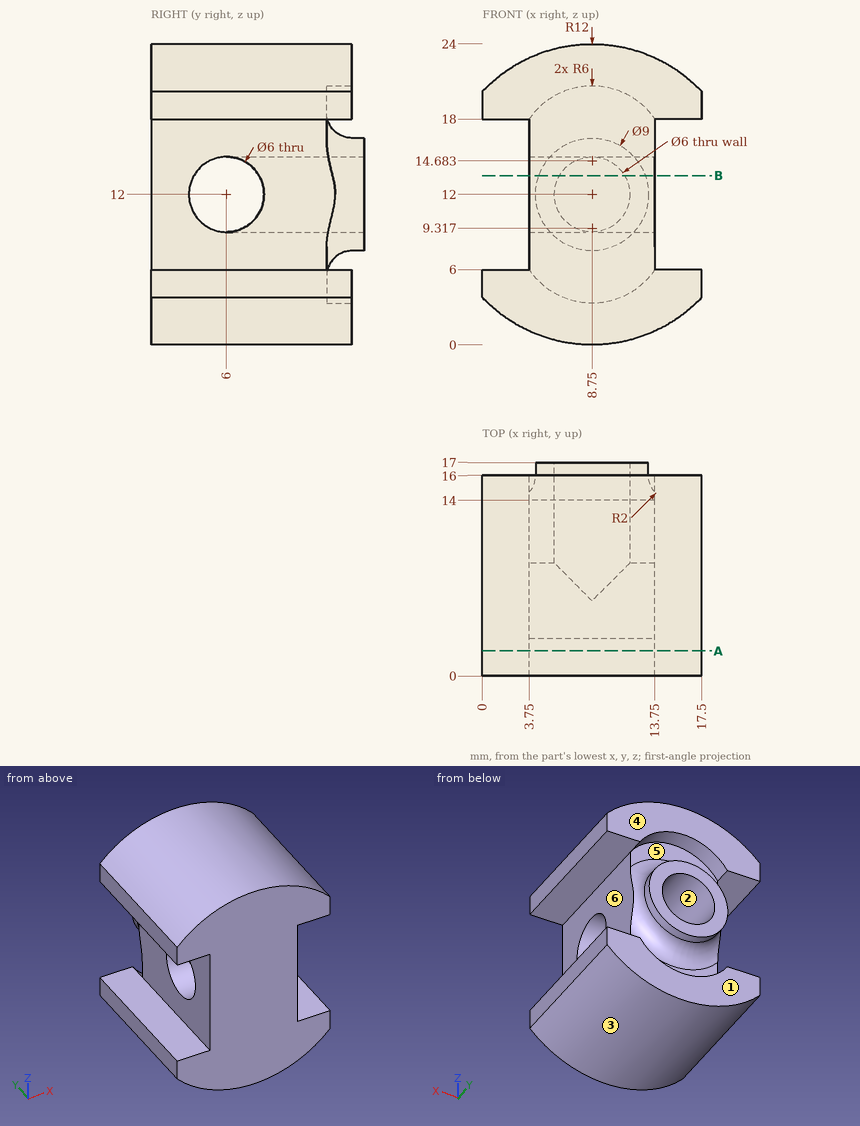
Input: dimensioned drawing with shaded views. Units: mm. Origin: part minimum x, y, z. A direction names the side the tool comes from. Coordinates: 2 decimals unless noted, no trailing zeros. Loops run counter-clockwise (first coordinate to the right, second up) from the corner with the lowest first, then second, coordinate; pieces in that order, holes last. Notation, with made-up numbers: (64.5, 88.5) -> (101.5, 88.5) arc R37 ccw to (101.5, 126.5) -> close; hole circle Ø3 at (-5.75, 88). An arc over 180 degrees is marked (long way). One line per item, written item: value. Start each with the question number.
Q1. Contact query for flat-ended pins moving along their axis: P1, Ø4, axis at y = 7.5, z = 10, coming from the +X side; P2, Ø5, axis at x = 7.5, z = 21.5, coming from the +Y side; P3, Ø5.5, axis at y = 6, z = 12, coming from the -X side; P4, Ø9.5, axis at y = 4.5, z = 13, coming from the -X side. Output: stop coordinate, or through.
Q2. Mould query, pull axis Z, two halves, no side actions, for the marked faces 1, 2 and 3. Classes: pulls with the +Z half, pulls with the -Z half, needs draft (parallel to the pull), parting line crosses it, or undercut.
Q3. Set-up query: the marked faces 4, 5 and 6. Return all of +Z, -Z, +X, -X, +Y, -Y with unobstructed straight access to the full face (end or side cutting, diameter ignored); none if empty.
Q4. Section query A-A, the plane y = 2. Return the cut outline in (x, z), and give its area (3 significant figures).
Q5. Section query B-B, the plane z = 13.5. Give the number of separate pieces and of enclosed holes in the cut face.
Q6. Line query: line 1 along Z through (x, y) = (8.75, 9); line 2 along X through (y, z) = (6, 8.25); line 3 along Y through (x, z) = (3, 19.5). Output: solid intervals per line, ascending.
Results:
1. P1: x = 13.75
1. P2: y = 16
1. P3: through
1. P4: x = 3.75
2. face 1: needs draft
2. face 2: undercut
2. face 3: pulls with the -Z half
3. face 4: +Z, +X, -X, +Y
3. face 5: +Y
3. face 6: +X, +Y, -Y
4. outline: (0, 3.79) arc R12 ccw to (17.5, 3.79) -> (17.5, 6) -> (13.75, 6) -> (13.75, 18) -> (17.5, 18) -> (17.5, 20.21) arc R12 ccw to (0, 20.21) -> (0, 18) -> (3.75, 18) -> (3.75, 6) -> (0, 6) -> close
4. area: 289 mm^2
5. separate pieces: 3
5. enclosed holes: 0
6. line 1: 0 to 9, 15 to 24
6. line 2: 3.75 to 13.75
6. line 3: 0 to 16
